Source: CAD feature listing. Evaluate the final solid. Frame: model axes, mm. A direction names the side the tool comes from. Give positions to 0.01 mm unless a question says otherwise; leave off trailing zeros. Write each loop counter-clockwise with the first axis right and the second up, starting at its lowest first coordinate (ties: lowest second). Pieces come first, ordered by that corner, then holes. Notation, with made-up numbers: (54, -6) - (67, -6) arc R19 ccw to (67, 7) - close; hole circle Ø7 at (-5, 12). An arc over 180 degrees is marked (long way). One line per question, with ' | ' between items. Start each with the question number.
(1) Section B-B, the plane y = 14. Return loops of the section in (x, z), plus the area to 3 significant figures.
(2) Section A-A, the plane z = -24. Return loops of the section in (x, y), plus the area to 3 significant figures.
(3) Section C-C, the plane x = -4. Return loops of the section in (y, z), plus the area to 4 significant figures.
(4) Ray query, line 1 (X direction, y = 9.25, z = -13); line 2 (Y direction, x = -4, z = -12); line 3 (X direction, y = 4.5, z = -20). Return the intervals inside material, ascending. Write a range as [from, to].
(5) Section D-D, the plane z = -2. Return loops of the section in (x, y), plus the area to 3 significant figures.
(6) Pin query (flat end, axial travel): pin 1 (4.5 mm diameter, centred on x = -16.5, y = 9, fed in from -Z); pin 2 (3 mm diameter, centred on x = 60, z = 1.5, fed in from -Y); pin 3 (2 mm diameter, centred on x = 30, y = 10, fed in from -Z). Return the tip coordinate at first contact, or that it passes through.
(7) Draft query along Y for faces 1 (the cylindrical face through (90.859, 8.874, -1.203)), 2 (the cylindrical face through (12, 15.5, 1.7)), 3 (the flat face through (30, 18, 1)). Return one class per face: +Y half, -Y half, draft (parallel to the pull), parting line (faces both ways), or undercut.
(8) Access query for faces 4 (the flat face through (62, 2, 2)), 5 (the flat face through (103, 9, -30)), 6 (the flat face through (92, 9, -17)). Directions: +Z, -Z, +X, -X, +Y, -Y. A direction counts if a zero-diameter tool reaches every point of the face in a straight line with its end or side. Return the directions, or none.
Autodesk Inventor part; units mm, degrees
ref_plane "YZ Plane" through (0, 0, 0) normal (1, 0, 0) x (0, 1, 0)
ref_plane "XZ Plane" through (0, 0, 0) normal (0, 1, 0) x (-1, 0, 0)
ref_plane "XY Plane" through (0, 0, 0) normal (0, 0, 1) x (1, 0, 0)
sketch "Sketch3" plane through (0, 0, 0) normal (0, 0, 1) x (1, 0, 0)
  line L0 (0, -3.6) -> (0, 21.6)
  line L1 (-49.2, 0) -> (141.2, 0)
  circle A0 centre (14, 14) radius 2.5
  line L2 (56.5, 11) -> (67.5, 11)
  line L3 (69.5, 9) -> (69.5, 4)
  line L4 (67.5, 2) -> (56.5, 2)
  line L5 (54.5, 4) -> (54.5, 9)
  line L6 (54.5, 11) -> (69.5, 2) construction
  line L7 (69.5, 11) -> (54.5, 2) construction
  arc A1 (69.5, 9) -> (67.5, 11) centre (67.5, 9) ccw
  arc A2 (67.5, 2) -> (69.5, 4) centre (67.5, 4) ccw
  arc A3 (54.5, 4) -> (56.5, 2) centre (56.5, 4) ccw
  arc A4 (56.5, 11) -> (54.5, 9) centre (56.5, 9) ccw
  line L8 (0, 18) -> (92, 18)
  line L9 (92, 18) -> (92, 0)
  line L10 (92, 0) -> (0, 0)
  line L11 (0, 0) -> (0, 18)
  line L12 (0, 18) -> (92, 0) construction
  line L13 (92, 18) -> (0, 0) construction
  line L14 (-22, 18) -> (0, 18)
  line L15 (0, 18) -> (0, 0)
  line L16 (0, 0) -> (-22, 0)
  line L17 (-22, 0) -> (-22, 18)
  line L18 (-22, 18) -> (0, 0) construction
  line L19 (0, 18) -> (-22, 0) construction
  line L20 (46, 18) -> (46, 0) construction
  line L21 (92, 18) -> (114, 18)
  line L22 (114, 18) -> (114, 0)
  line L23 (114, 0) -> (92, 0)
  line L24 (92, 0) -> (92, 18)
  line L25 (92, 18) -> (114, 0) construction
  line L26 (114, 18) -> (92, 0) construction
  point P0 (0, 0)
  point P1 (62, 6.5)
  point P2 (54.5, 6.5)
  point P3 (46, 9)
  point P4 (-11, 9)
  point P5 (103, 9)
  point P6 (-22, 0)
  point P7 (114, 0)
  point P8 (92, 18)
  point P9 (92, 0)
  point P10 (96, 9)
  point P11 (108.5, 9)
  point P12 (-4, 9)
  point P13 (-16.5, 9)
  dimension "d26" = 5
  dimension "d29" = 15
  dimension "d30" = 9
  dimension "d31" = 2
  dimension "d34" = 92
  dimension "d35" = 18
  dimension "d36" = 22
  dimension "d37" = 18
  dimension "d38" = 22
  dimension "d39" = 18
  dimension "d41" = 14
  dimension "d42" = 14
  dimension "d56" = 62
  dimension "d57" = 6.5
  dimension "d60" = 50
  dimension "d61" = 62.5
  dimension "d62" = 9
extrude "Extrusion4" add sketch "Sketch3" along normal blind 3.5
extrude "Extrusion5" add sketch "Sketch3" against normal blind 30 contours L1 L17 L14 L0 | L9 L21 L22 L1
hole "Hole1" at (96, 9, 0) at (108.5, 9, 0) at (-4, 9, 0) at (-16.5, 9, 0) direction (0, 0, -1) diameter 5 end through all both
fillet "Fillet1" radius 4 2 edges at (0, 9, 0) (92, 9, 0)
properties part number "camera_holder"
Check sheet entries:
1) outline: (-22, -30) - (0, -30) - (0, -4) arc R4 cw to (4, 0) - (11.5, 0) - (11.5, 3.5) - (-22, 3.5) - close; (16.5, 0) - (88, 0) arc R4 cw to (92, -4) - (92, -30) - (114, -30) - (114, 3.5) - (16.5, 3.5) - close | area: 1,790 mm²
2) outline: (-22, 0) - (0, 0) - (0, 18) - (-22, 18) - close; (92, 0) - (114, 0) - (114, 18) - (92, 18) - close; hole circle Ø5 at (-16.5, 9); hole circle Ø5 at (-4, 9); hole circle Ø5 at (96, 9); hole circle Ø5 at (108.5, 9) | area: 713 mm²
3) outline: (0, -30) - (6.5, -30) - (6.5, 3.5) - (0, 3.5) - close; (11.5, -30) - (18, -30) - (18, 3.5) - (11.5, 3.5) - close | area: 435.5 mm²
4) line 1: [-22, -18.99], [-14.01, -6.49], [-1.51, 0], [92, 93.51], [98.49, 106.01], [110.99, 114] | line 2: [0, 6.5], [11.5, 18] | line 3: [-22, 0], [92, 114]
5) outline: (-22, 0) - (0.54, 0) - (0.54, 18) - (-22, 18) - close; (91.46, 0) - (114, 0) - (114, 18) - (91.46, 18) - close; hole circle Ø5 at (-16.5, 9); hole circle Ø5 at (-4, 9); hole circle Ø5 at (96, 9); hole circle Ø5 at (108.5, 9) | area: 733 mm²
6) pin 1: through | pin 2: y = 0 | pin 3: z = 0
7) face 1: draft | face 2: undercut | face 3: +Y half
8) face 4: +Z, -Z | face 5: -Z, +X, -X, +Y, -Y | face 6: -Z, +Y, -Y
